from build123d import *

# Parameters (mm, degrees)
F0_W     = 15
F0_H     = 8
F1_DEPTH = 15
F1_TAPER = 3
F2_R     = 2.5
F3_DEPTH = 5
F4_R     = 1
F5_R     = 1.5
F6_DEPTH = 3
F7_R     = 1.5
F8_DEPTH = 3


with BuildPart() as f1:
    # F0 (on Top) → F1 (new body)
    with BuildSketch(Plane.XY):
        Rectangle(F0_W, F0_H)
    extrude(amount=F1_DEPTH, taper=F1_TAPER)

    # F2 (on face) → F3 (join)
    with BuildSketch(Plane.XY.offset(15)):
        Circle(F2_R)
    extrude(amount=F3_DEPTH)

    # F4
    f4_edges = [f1.edges().sort_by_distance(p)[0] for p in [
        (-7.106942, -3.606942, 7.5),
        (0, -3.213883, 15),
        (7.106942, -3.606942, 7.5),
        (6.713883, 0, 15),
        (7.106942, 3.606942, 7.5),
        (-6.713883, 0, 15),
        (-7.106942, 3.606942, 7.5),
    ]]
    fillet(f4_edges, radius=F4_R)

    # F5 (on face) → F6 (cut)
    with BuildSketch(Plane(origin=(-7.4794571076, 0, 0.3919817373), x_dir=(0, -1, 0), z_dir=(-0.9986295348, 0, 0.0523359562))):
        with Locations((0, 10.6777304862)):
            Circle(F5_R)
    extrude(amount=-F6_DEPTH, mode=Mode.SUBTRACT)

    # F7 (on face) → F8 (cut)
    with BuildSketch(Plane(origin=(7.4794571076, 0, 0.3919817373), x_dir=(0, 1, 0), z_dir=(0.9986295348, 0, 0.0523359562))):
        with Locations((0, 10.7058982886)):
            Circle(F7_R)
    extrude(amount=-F8_DEPTH, mode=Mode.SUBTRACT)


solid = f1.part
Could you check a few things on this model? Use its own coordinates, in mm. A direction names the side the tool comes from. Give positions to 0.01 mm unless a question says otherwise; leave off trailing zeros. Order: outer loops, then holes, each group sorted by start corner. A loop starts at its lowest first (then second) coordinate and runs counter-clockwise, first axis right, second up.
1. Will these pins go through, and if not, where does the flat tip stop? P1, Ø3, axis at x = -5.5, z = 11, coming from the -Y side; P2, Ø3, axis at x = 3.5, y = -1.5, coming from the +Z side; P3, Ø1.5, axis at y = -2.5, z = 15.5, coming from the +X side (3 decimals).
2. Suppose I cut it at B-B (z = 15.25). List the corners of the cut face in (x, y) for me.
3. Suppose I cut it at C-C (x = 3.5). List the corners of the cut face in (y, z) for me.
4. We'd pull the mould along Z, two halves only. Please class faces 1 (the flat face through (0.091, -3.636, 6.947)), 2 (the flat face through (0, 0, 0)), 3 (the cylindrical face through (5.512, 0.692, 9.677)): pulls with the +Z half, pulls with the -Z half, needs draft (parallel to the pull), parting line crosses it, or undercut.
5. For faces 4 (the cylindrical face through (3.44, -2.96, 14.72)), 5 (the flat face through (0, 0, 20)), 6 (the cylindrical face through (-0.54, -2.44, 17.46)), which set-ups out of +Z, -Z, +X, -X, +Y, -Y let a thin tool reach every point of the face, with its end or its side?
6. I need wall thicknesses on L1, parallel to Z at x = 3.75, y = -1.25; L2, parallel to Z at x = 5, y = 1; L3, parallel to Y at x = 3.5, z = 1.25. Which ranges of each line are inside material? Lowest first, please.
7. Suppose I cut it at A-A (y = 0). List the corners of the cut face in (x, z) for me, plus the area to 3 significant figures.
Solved:
1. P1: stops at y = -3.5
1. P2: stops at z = 20
1. P3: stops at x = 6.405
2. outline: circle Ø5 at (0, 0)
3. outline: (-4, 0) - (4, 0) - (3.21, 15) - (-2.26, 15) arc R1 ccw to (-3.26, 14.05) - close
4. face 1: pulls with the +Z half
4. face 2: pulls with the -Z half
4. face 3: undercut
5. face 4: +Z, +X, -Y
5. face 5: +Z, +X, -X, +Y, -Y
5. face 6: +Z
6. L1: z = 0 to 15
6. L2: z = 0 to 9.86, 12.1 to 15
6. L3: y = -3.93 to 3.93
7. outline: (-7.5, 0) - (7.5, 0) - (7, 9.59) - (4, 9.43) - (3.84, 12.42) - (6.84, 12.58) - (6.76, 14.05) arc R1 ccw to (5.76, 15) - (2.5, 15) - (2.5, 20) - (-2.5, 20) - (-2.5, 15) - (-5.76, 15) arc R1 ccw to (-6.76, 14.05) - (-6.84, 12.55) - (-3.85, 12.4) - (-4, 9.4) - (-7, 9.56) - close
7. area: 220 mm2
